```python
from build123d import *

# Parameters (mm, degrees)
SKETCH_1_W      = 22.86
SKETCH_1_H      = 8.5
EXTRUDE_1_DEPTH = 2.5
SKETCH_2_W      = 0.6
SKETCH_2_H      = 0.4
EXTRUDE_2_DEPTH = 3


with BuildPart() as part:
    # Эскиз1 → Бобышка-Вытянуть1 (new body)
    with BuildSketch(Plane(origin=(0, 0, 0), x_dir=(1, 0, 0), z_dir=(0, 1, 0))):
        Rectangle(SKETCH_1_W, SKETCH_1_H)
    extrude(amount=EXTRUDE_1_DEPTH)

    # Эскиз2 → Бобышка-Вытянуть2 (add)
    with BuildSketch(Plane.XY.offset(4.25)):
        with Locations((-7.62, 1.25)):
            Rectangle(SKETCH_2_W, SKETCH_2_H)
        with Locations((-10.16, 1.25)):
            Rectangle(SKETCH_2_W, SKETCH_2_H)
        with Locations((-5.08, 1.25)):
            Rectangle(SKETCH_2_W, SKETCH_2_H)
        with Locations((-2.54, 1.25)):
            Rectangle(SKETCH_2_W, SKETCH_2_H)
        with Locations((0, 1.25)):
            Rectangle(SKETCH_2_W, SKETCH_2_H)
        with Locations((2.54, 1.25)):
            Rectangle(SKETCH_2_W, SKETCH_2_H)
        with Locations((5.08, 1.25)):
            Rectangle(SKETCH_2_W, SKETCH_2_H)
        with Locations((7.62, 1.25)):
            Rectangle(SKETCH_2_W, SKETCH_2_H)
        with Locations((10.180976984, 1.25)):
            Rectangle(SKETCH_2_W, SKETCH_2_H)
    extrude(amount=EXTRUDE_2_DEPTH)


solid = part.part
```
CAD build for the part. Positions are in the model's coordinates, mm. Coordinates: 2 decimals unless noted, no trailing zeros. Order: outer loops, then holes, each group sorted by start corner. A loop starts at its lowest first (then second) coordinate and runs counter-clockwise, first axis right, second up. Notation, with made-up numbers: (50.25, 15) -> (89.25, 15) arc R19 ccw to (89.25, 25) -> close; hole circle Ø1 at (33.5, 76). An arc over 180 degrees is marked (long way). Use one line per item in the form item = value. Start each with the question number.
1) Band-saw the part on A-A on x = 0. Give the cut face in (y, z).
2) Band-saw the part on C-C on x = 3.5. Give the cut face in (y, z).
3) Band-saw the part on B-B on z = 5.5. State how many separate pieces and enclosed holes the cut face has, then the cut area to 3 significant figures.
4) Drop flat-ended pins along their axis: pin 1 (0.7 mm diameter, centred on x = 7.5, z = 6, fed in from +Y); pin 2 (0.5 mm diameter, centred on x = 10, z = 6.5, fed in from -Y); pin 3 (5 mm diameter, centred on x = 2, z = -1, fed in from -Y); pin 4 (1 mm diameter, centred on x = 0.5, y = 0.5, fed in from +Z). Give the stop position or say it passes through.
5) Drill centre lines: L1, parallel to Z at x = -4.75, y = 1.35; L2, parallel to Y at x = -7.5, z = 6.5. Where is each one in solid material? Low to high. Write a range as [from, to].
Entries:
q1.outline = (0, -4.25) -> (2.5, -4.25) -> (2.5, 4.25) -> (1.45, 4.25) -> (1.45, 7.25) -> (1.05, 7.25) -> (1.05, 4.25) -> (0, 4.25) -> close
q2.outline = (0, -4.25) -> (2.5, -4.25) -> (2.5, 4.25) -> (0, 4.25) -> close
q3.separate_pieces = 9
q3.enclosed_holes = 0
q3.area = 2.16 mm2
q4.pin_1 = 1.45
q4.pin_2 = 1.05
q4.pin_3 = 0
q4.pin_4 = 4.25
q5.L1 = [-4.25, 4.25]
q5.L2 = [1.05, 1.45]
